```python
from build123d import *

# Parameters (mm, degrees)
ESQUISSE1_R        = 15
BOSS_EXTRU_1_DEPTH = 5
ESQUISSE5_R        = 20
ESQUISSE5_R_2      = 15
BOSS_EXTRU_2_DEPTH = 2
CHANFREIN2_SIZE    = 2
CHANFREIN2_SIZE_2  = 3.464101615
CONG_1_R           = 2


with BuildPart() as part:
    # Esquisse1 → Boss.-Extru.1 (new body)
    with BuildSketch(Plane.XY):
        with BuildLine():
            Line((-10, 17.320508076), (-10, 22))
            Line((-10, 22), (-15, 22))
            Line((-15, 22), (-17.030050858, 10.487009478))
            ThreePointArc((-17.030050858, 10.487009478), (-20, 0), (-17.030050858, -10.487009478))
            Line((-17.030050858, -10.487009478), (-15, -22))
            Line((-15, -22), (-10, -22))
            Line((-10, -22), (-10, -17.320508076))
            ThreePointArc((-10, -17.320508076), (0, -20), (10, -17.320508076))
            Line((10, -17.320508076), (10, -22))
            Line((10, -22), (15, -22))
            Line((15, -22), (17.030050858, -10.487009478))
            ThreePointArc((17.030050858, -10.487009478), (18.403131111, -7.831013044), (19.364916731, -5))
            Line((19.364916731, -5), (20, -5))
            Line((20, -5), (20, 5))
            Line((20, 5), (19.364916731, 5))
            ThreePointArc((19.364916731, 5), (18.403131111, 7.831013044), (17.030050858, 10.487009478))
            Line((17.030050858, 10.487009478), (15, 22))
            Line((15, 22), (10, 22))
            Line((10, 22), (10, 17.320508076))
            ThreePointArc((10, 17.320508076), (0, 20), (-10, 17.320508076))
        make_face()
        Circle(ESQUISSE1_R, mode=Mode.SUBTRACT)
    extrude(amount=BOSS_EXTRU_1_DEPTH)

    # Esquisse5 → Boss.-Extru.2 (add)
    with BuildSketch(Plane.XY.offset(5)):
        Circle(ESQUISSE5_R)
        Circle(ESQUISSE5_R_2, mode=Mode.SUBTRACT)
    extrude(amount=BOSS_EXTRU_2_DEPTH)

    # Chanfrein2
    # the kernel refuses this chamfer: 3.464101615, 2 mm, written as the material it takes off along each edge
    with BuildSketch(Plane(origin=(0, 0, 7), x_dir=(1, 0, 0), z_dir=(0, -1, 0))) as chanfrein2_piece_1:
        Polygon((20, -CHANFREIN2_SIZE), (20 - CHANFREIN2_SIZE_2, 0), (20, 0), align=None)
    revolve(axis=Axis((0, 0, 7), (0, 0, 1)), mode=Mode.SUBTRACT)

    # Congé1
    cong_1_edges = [part.edges().sort_by_distance(p)[0] for p in [
        (12.5, -22, 5),
        (-12.5, -22, 5),
        (12.5, 22, 5),
        (-12.5, 22, 5),
    ]]
    fillet(cong_1_edges, radius=CONG_1_R)


solid = part.part
```
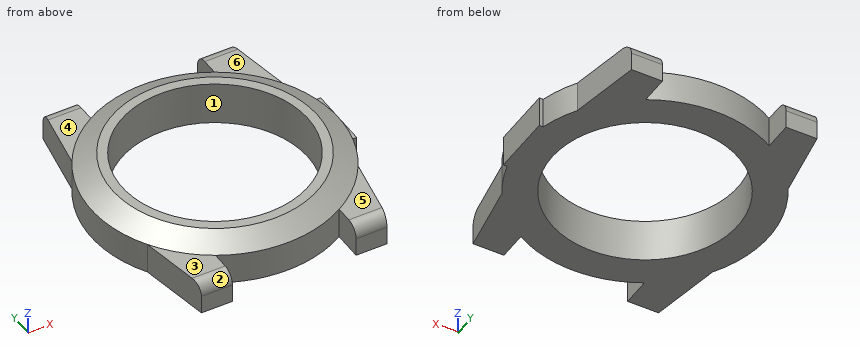
The model under review builds one solid part; all positions refer to its coordinate system, in mm. Face numbers are marked on the shaded views. A direction names the side the tool comes from. Coordinates: 2 decimals unless noted, no trailing zeros. Order: outer loops, then holes, each group sorted by start corner. A loop starts at its lowest first (then second) coordinate and runs counter-clockwise, first axis right, second up. Notation, with made-up numbers: M -32,83.25 L 16,83.25 A12 cw 16,98.25 Z; hole C 26,-37.75 d3. An arc over 180 degrees is marked long. One line per question, with ' | ' between items.
(1) For probe 1 along Y at (x, z) = (0, 2); probe 2 along X at (y, z) = (-17.5, 3.5); probe 3 along Y at (x, z) = (11.5, 3.5), list the stretches that pass through material, from the lowest coordinate up. Write a range as from..to.
Geometry results:
probe 1: y = -20..-15, 15..20 | probe 2: x = -15.79..-10, -9.68..9.68, 10..15.79 | probe 3: y = -21.94..-9.63, 9.63..21.94
(2) Add section C-C, the plane z = 4. Write out the cut boundary in (x, y), then the cut area to 3 significant figures.
Geometry results:
outline: M -17.03,-10.49 L -15.05,-21.73 L -10,-21.73 L -10,-17.32 A20 ccw 10,-17.32 L 10,-21.73 L 15.05,-21.73 L 17.03,-10.49 A20 ccw 19.36,-5 L 20,-5 L 20,5 L 19.36,5 A20 ccw 17.03,10.49 L 15.05,21.73 L 10,21.73 L 10,17.32 A20 ccw -10,17.32 L -10,21.73 L -15.05,21.73 L -17.03,10.49 A20 ccw Z; hole C 0,0 d30 | area: 711 mm²
(3) Add section A-A, the plane x = 0. Write out the cut boundary in (y, z), then the cut area to 3 significant figures.
Geometry results:
outline: M -20,0 L -15,0 L -15,7 L -16.54,7 L -20,5 Z; M 15,0 L 20,0 L 20,5 L 16.54,7 L 15,7 Z | area: 63.1 mm²
(4) Machinability: for the marked faces 4, 5 and 6, which of the approach directions +Z, -Z, +X, -X, +Y, -Y give a long, thin tool a straight path to every point of the face, cutting with its end or side? Answer none if there is none.
Geometry results:
face 4: +Z, -X, +Y | face 5: +Z, +X, -Y | face 6: +Z, +X, +Y
(5) The part is to be moulded in two halves that separate along Y. For the marked faces 1, 2 and 3, say which applies: +Y half, -Y half, draft (parallel to the pull), parting line (faces both ways), or undercut.
Geometry results:
face 1: undercut | face 2: -Y half | face 3: draft
(6) Insertion check: pin 1 (24 mm diameter, centred on x = 0, y = 0, fed in from -Z); pin 2 (2 mm diameter, centred on x = 12.5, y = -15, fed in from +Z); pin 3 (0.7 mm diameter, centred on x = 20, z = 3, fed in from +Y); pin 4 (3.5 mm diameter, centred on y = -20.5, z = 1.5, fed in from -X). Each pin has a flat end and moves straight along its axis. Give the tip position at first contact, or say it passes through.
Geometry results:
pin 1: passes through | pin 2: stops at z = 5.85 | pin 3: stops at y = 5 | pin 4: stops at x = -15.57
(7) Add section B-B, the plane z = 1. Write out the cut boundary in (x, y).
Geometry results:
outline: M -17.03,-10.49 L -15,-22 L -10,-22 L -10,-17.32 A20 ccw 10,-17.32 L 10,-22 L 15,-22 L 17.03,-10.49 A20 ccw 19.36,-5 L 20,-5 L 20,5 L 19.36,5 A20 ccw 17.03,10.49 L 15,22 L 10,22 L 10,17.32 A20 ccw -10,17.32 L -10,22 L -15,22 L -17.03,10.49 A20 ccw Z; hole C 0,0 d30
